from build123d import *

# Parameters (mm, degrees)
F1_DEPTH    = 15
F2_R        = 0.5
F3_T1_DEPTH = 66.9437702684
F4_SIZE2    = 2.5
F4_SIZE     = 10


# Not quite as in the source:
# - a fillet or chamfer that OpenCascade refuses, or shapes differently, is made with other operations: its cross-section is extruded or revolved along the edge and cut away or added


with BuildPart() as f1:
    # F0 (on Top) → F1 (new body)
    with BuildSketch(Plane.XY):
        Polygon((25.5, 20), (-25.5, 20), (-25.5, -20), (-19.5, -20), (-19.25, -14), (-19.25, 14), (19.25, 14), (19.25, -14), (19.25, -20), (25.5, -20), align=None)
    extrude(amount=F1_DEPTH)

    # F2
    f2_edges = [f1.edges().sort_by_distance(p)[0] for p in [
        (-19.25, 14, 7.5),
        (19.25, 14, 7.5),
        (-25.5, 20, 7.5),
        (25.5, 20, 7.5),
    ]]
    fillet(f2_edges, radius=F2_R)

    # F3: chamfer of 10 x 2.5 on 1 edges, made by hand

    # F3_s2 → F3_t1 (cut)
    with BuildSketch(Plane.XY.offset(-25.9718851342)):
        Polygon((-22, -20), (-19.0836945529, -10.0086692691), (-19.5, -20), align=None)
    extrude(amount=F3_T1_DEPTH, mode=Mode.SUBTRACT)

    # F4
    f4_edges = [f1.edges().sort_by_distance(p)[0] for p in [
        (19.25, -20, 7.5),
    ]]
    f4_side = f1.faces().sort_by_distance((19.25, -3.25, 7.5))[0]
    chamfer(f4_edges, length=F4_SIZE, length2=F4_SIZE2, reference=f4_side)


solid = f1.part
Geometry check sheet. Reference: the model listing, model coordinates, mm. A direction names the side the tool comes from. Coordinates: 2 decimals unless noted, no trailing zeros. Order: outer loops, then holes, each group sorted by start corner. A loop starts at its lowest first (then second) coordinate and runs counter-clockwise, first axis right, second up. Notation, with made-up numbers: M -27,77.25 L 20,77.25 A34 cw 20,107.25 Z; hole C 10.25,-14.75 d5. An arc over 180 degrees is marked long. Use CSV: the item, a comma, the result in double quotes.
Item 1: Cross-section at C-C on x = 16.5. Record the cut outline in (y, z).
Returned:
outline,"M 14,0 L 20,0 L 20,15 L 14,15 Z"
Item 2: Cross-section at D-D on y = -16.5. Record the cut outline in (x, z) (3 decimals), then the cut area to 3 significant figures.
Returned:
outline,"M -25.5,0 L -20.978,0 L -20.978,15 L -25.5,15 Z; M 20.875,0 L 25.5,0 L 25.5,15 L 20.875,15 Z"
area,"137 mm2"
Item 3: Cross-section at A-A on y = 8.5. Record the cut outline in (x, z).
Returned:
outline,"M -25.5,0 L -19.25,0 L -19.25,15 L -25.5,15 Z; M 19.25,0 L 25.5,0 L 25.5,15 L 19.25,15 Z"
Item 4: Gauge pin test, flat ends, axial feed: pin 1 Ø7.5 at (x, z) = (9, 4) entering from -Y; pin 2 Ø12 at (x, y) = (-18, 5.5) entering from -Z. Record the tip position at first contact, or that the pin passes through.
Returned:
pin 1,"stops at y = 14"
pin 2,"stops at z = 0"
Item 5: Mould release check, pull along X, two halves, no side actions. Record for faces 1 (the flat face through (0, 14, 7)), 2 (the flat face through (-25.5, 0, 7)), 3 (the flat face through (0, 20, 7)), 4 (the flat face through (19.25, 2, 7)): pulls with the +X half, pulls with the -X half, needs draft (parallel to the pull), parting line crosses it, or undercut.
Returned:
face 1,"undercut"
face 2,"pulls with the -X half"
face 3,"needs draft"
face 4,"undercut"
Item 6: Thickness scan on line 1 along X through (y, z) = (10, 11.25); line 2 along Y through (x, z) = (10, 13.5); line 3 along X through (y, z) = (-11, 4.25). Record the ranges inside material, lowest first.
Returned:
line 1,"x = -25.5 to -19.25, 19.25 to 25.5"
line 2,"y = 14 to 20"
line 3,"x = -25.5 to -19.37, 19.5 to 25.5"
Item 7: Tool access check on faces 5 (the flat face through (-19.25, 1, 7)), 6 (the flat face through (-2, 15, 0)). Record the directions out of +Z, -Z, +X, -X, +Y, -Y that give a thin tool (end or side, any length) a straight path to the whole face; none if there is none.
Returned:
face 5,"+Z, -Z, -Y"
face 6,"-Z, +X, -X, +Y, -Y"
Item 8: Cross-section at B-B on z = 3.75. Record the cut outline in (x, y).
Returned:
outline,"M -25.5,-20 L -22,-20 L -19.25,-10.58 L -19.25,13.5 A0.5 cw -18.75,14 L 18.75,14 A0.5 cw 19.25,13.5 L 19.25,-10 L 21.75,-20 L 25.5,-20 L 25.5,19.5 A0.5 ccw 25,20 L -25,20 A0.5 ccw -25.5,19.5 Z"
